Input: part model. Units: mm. Frame: model coordinates. A direction names the side the tool comes from. Coordinates: 2 decimals unless noted, no trailing zeros. Loops run counter-clockwise (first coordinate to the right, second up) from the corner with the lowest first, then second, coordinate; pieces in that order, holes last.
Item 1: Section C-C on y = -109. Return loops of the section in (x, z), and give its area (3 significant figures).
Item 2: Section D-D on x = 26. Return loops of the section in (y, z).
Item 3: Contact query for flat-ended pins moving along their axis: P1, Ø2, axis at x = 36, y = -79, coming from the -Z side; P2, Ø10, axis at x = 197, y = -18, coming from the +Z side; P3, Ø20, axis at x = 191, y = -52, coming from the -Z side. Output: stop coordinate, or through.
Item 4: Reachability of faces 4 (the flat face through (75, -14, 77.19)), 5 (the cylindrical face through (136.355, -22.002, 64.312)), 6 (the flat face through (44, -66, 49.25)) from +Z, -Z, +X, -X, +Y, -Y: full face, straight path, thin tool, end or side. Return the list, or none.
Item 5: Section B-B on z = 32. Return loops of the section in (x, y), and give its area (3 significant figures).
Item 6: Ray query, line 1 along X through (y, z) = (5, 7); line 2 along Y through (x, z) = (165, -25); line 3 along Y through (x, z) = (64, 36.5). Return the intervals inside material, ascending.
Item 7: Pull-direction query (X, two-part tool) for faces 1 (the flat face through (113, -121.422, 1)), 2 (the flat face through (176, -13, 77.19)), 3 (the flat face through (2.54, -56, 3)); classes: released by +X, released by -X, zero draft, split by the parting line, or undercut.
Item 8: Section A-A on z = 68.5. Return loops of the section in (x, y), and give its area (3 significant figures).
```python
from build123d import *

# Parameters (mm, degrees)
F0_W      = 138.6799942702
F0_H      = 97.2796790302
F1_DEPTH  = 228.6
F2_T      = -2.54
F3_R      = 33.1351902141
F3_R_2    = 22.3789539676
F4_DEPTH  = 88.9
F5_R      = 31.365179226
F5_R_2    = 22.8340375073
F6_DEPTH  = 88.9
F7_R      = 32.921040163
F7_R_2    = 24.2040309483
F8_DEPTH  = 88.9
F9_R      = 12.840995734
F9_R_2    = 12.8521164222
F9_R_3    = 12.7516607916
F9_R_4    = 14.5420806557
F9_R_5    = 17.1317992696
F9_R_6    = 16.2815585051
F9_R_7    = 13.9618543487
F9_R_8    = 16.2927152835
F10_DEPTH = 25.4


with BuildPart() as f1:
    # F0 (on Right) → F1 (new body)
    with BuildSketch(Plane.YZ):
        with Locations((-54.6218389645, 3.1497571617)):
            Rectangle(F0_W, F0_H)
    extrude(amount=F1_DEPTH)

    # F2
    f2_openings = [f1.faces().sort_by_distance(p)[0] for p in [
        (114.3, -54.621839, -45.490082),
    ]]
    offset(amount=F2_T, openings=f2_openings)

    # F3 (on face) → F4 (join)
    with BuildSketch(Plane(origin=(0, 0, 49.2495966768), x_dir=(1, 0, 0), z_dir=(0, 0, -1))):
        with Locations((43.8807010651, 65.2723014355)):
            Circle(F3_R)
        with Locations((43.8807010651, 65.2723014355)):
            Circle(F3_R_2, mode=Mode.SUBTRACT)
    extrude(amount=F4_DEPTH)

    # F5 (on face) → F6 (join)
    with BuildSketch(Plane(origin=(0, 0, 49.2495966768), x_dir=(1, 0, 0), z_dir=(0, 0, -1))):
        with Locations((109.2752963305, 67.5403177738)):
            Circle(F5_R)
        with Locations((109.2752963305, 67.5403177738)):
            Circle(F5_R_2, mode=Mode.SUBTRACT)
    extrude(amount=F6_DEPTH)

    # F7 (on face) → F8 (join)
    with BuildSketch(Plane(origin=(0, 0, 49.2495966768), x_dir=(1, 0, 0), z_dir=(0, 0, -1))):
        with Locations((174.669906497, 65.6502991915)):
            Circle(F7_R)
        with Locations((174.669906497, 65.6502991915)):
            Circle(F7_R_2, mode=Mode.SUBTRACT)
    extrude(amount=F8_DEPTH)

    # F9 (on face) → F10 (join)
    with BuildSketch(Plane.XY.offset(51.7895966768)):
        with Locations((31.5596684813, -13.9110339805)):
            Circle(F9_R)
        with Locations((74.8604610562, -14.4456122071)):
            Circle(F9_R_2)
        with Locations((124.5761811733, -17.1185005456)):
            Circle(F9_R_3)
        with Locations((175.8956313133, -13.3764576167)):
            Circle(F9_R_4)
        with Locations((174.5792776346, -76.9741907716)):
            Circle(F9_R_5)
        with Locations((123.3455315232, -68.3407709002)):
            Circle(F9_R_6)
        with Locations((77.4572491646, -59.7661323845)):
            Circle(F9_R_7)
        with Locations((25.5353599787, -66.1121979356)):
            Circle(F9_R_8)
    extrude(amount=F10_DEPTH)


solid = f1.part
```
Results found:
1. outline: (0, -45.49) - (2.54, -45.49) - (2.54, 49.25) - (226.06, 49.25) - (226.06, -45.49) - (228.6, -45.49) - (228.6, 51.79) - (0, 51.79) - close
1. area: 1,060 mm2
2. outline: (-123.96, -45.49) - (-121.42, -45.49) - (-121.42, 49.25) - (-93.17, 49.25) - (-93.17, -39.65) - (-78.73, -39.65) - (-78.73, 49.25) - (-51.82, 49.25) - (-51.82, -39.65) - (-37.38, -39.65) - (-37.38, 49.25) - (12.18, 49.25) - (12.18, -45.49) - (14.72, -45.49) - (14.72, 51.79) - (-2.34, 51.79) - (-2.34, 77.19) - (-25.49, 77.19) - (-25.49, 51.79) - (-49.83, 51.79) - (-49.83, 77.19) - (-82.4, 77.19) - (-82.4, 51.79) - (-123.96, 51.79) - close
3. P1: stops at z = 49.25
3. P2: stops at z = 51.79
3. P3: stops at z = -39.65
4. face 4: +Z, +X, -X, +Y, -Y
4. face 5: +Z
4. face 6: -Z
5. outline: (0, -123.96) - (228.6, -123.96) - (228.6, 14.72) - (0, 14.72) - close; circle Ø66.27 at (43.88, -65.27); circle Ø62.73 at (109.28, -67.54); circle Ø65.84 at (174.67, -65.65); hole (2.54, -121.42) - (226.06, -121.42) - (226.06, 12.18) - (2.54, 12.18) - close; hole circle Ø44.76 at (43.88, -65.27); hole circle Ø45.67 at (109.28, -67.54); hole circle Ø48.41 at (174.67, -65.65)
5. area: 6,730 mm2
6. line 1: x = 0 to 2.54, 226.06 to 228.6
6. line 2: y = -123.96 to -121.42, -97.12 to -87.84, -43.46 to -34.18, 12.18 to 14.72
6. line 3: y = -123.96 to -121.42, -91.6 to -75.07, -55.47 to -38.94, 12.18 to 14.72
7. face 1: undercut
7. face 2: zero draft
7. face 3: undercut
8. outline: circle Ø32.59 at (25.54, -66.11); circle Ø25.68 at (31.56, -13.91); circle Ø25.7 at (74.86, -14.45); circle Ø27.92 at (77.46, -59.77); circle Ø32.56 at (123.35, -68.34); circle Ø25.5 at (124.58, -17.12); circle Ø34.26 at (174.58, -76.97); circle Ø29.08 at (175.9, -13.38)
8. area: 5,410 mm2
